Verification items for the finished model (mm, model axes). Coordinates: 2 decimals unless noted, no trailing zeros. Loops run counter-clockwise (first coordinate to the right, second up) from the corner with the lowest first, then second, coordinate; pieces in that order, holes last. Notation, with made-up numbers: (11.5, -29.5) - (49.5, -29.5) arc R34 cw to (49.5, 0.5) - close; hole circle Ø10 at (42.25, -5.5). An arc over 180 degrees is marked (long way). Answer as CSV lines item,"result". Start each with the question number.
1. Release check for a two-part mould opening along Y. For faces 1 (the cylindrical face through (265.014, -0.574, 1.972)), 2 (the cylindrical face through (-9.69, 0.42, 1.97)), 3 (the flat face through (125, 0, 4)) record: pulls with the +Y half, pulls with the -Y half, needs draft (parallel to the pull), parting line crosses it, or undercut.
2. Material ranges on line 1 (X direction, y = 0, z = 1.8); line 2 (X direction, y = 3, z = 2.95); line 3 (X direction, y = 8.5, z = 1), recorded low to high. Write a range as [from, to].
3. Cross-section at C-C (x = 250). Enter the section's corners in (y, z).
4. Cross-section at D-D (x = 136.5). Enter the section's corners in (y, z), plus the area to 3 significant figures.
5. Cross-section at A-A (x = 0). Enter the section's corners in (y, z).
6. Cross-section at B-B (z = 2.2). Enter the section's corners in (x, y).
7. Gauge pin test, flat ends, axial feed: P1, Ø2, axis at y = -2, z = 2.5, coming from the -X side; P2, Ø1, axis at y = 10.5, z = 0.5, coming from the +X side; P3, Ø1, axis at y = -8.5, z = 3.5, coming from the +X side. Record the tip position at first contact, or that the pin passes through.
```python
from build123d import *

# Parameters (mm, degrees)
SKETCH_1_R          = 9.7
SKETCH_1_R_2        = 1.5
EXTRUDE_1_DEPTH     = 4
SKETCH_3_R          = 0.8
CUT_EXTRUDE_1_DEPTH = 10


with BuildPart() as part:
    # 草图1 → 凸台-拉伸1 (new body)
    with BuildSketch(Plane.XY):
        with BuildLine():
            ThreePointArc((12.718684308, 6), (-14.062891969, 0), (12.718684308, -6))
            Line((12.718684308, -6), (236.224480753, -6))
            ThreePointArc((236.224480753, -6), (265.02547605, 0), (236.224480753, 6))
            Line((236.224480753, 6), (127.47158253, 6))
            ThreePointArc((127.47158253, 6), (124.47158253, 9), (121.47158253, 6))
            Line((121.47158253, 6), (12.718684308, 6))
        make_face()
        Circle(SKETCH_1_R, mode=Mode.SUBTRACT)
        with Locations((250, 0)):
            Circle(SKETCH_1_R, mode=Mode.SUBTRACT)
        with Locations((124.47158253, 6)):
            Circle(SKETCH_1_R_2, mode=Mode.SUBTRACT)
    extrude(amount=EXTRUDE_1_DEPTH)

    # 草图3 → 切除-拉伸1 (cut)
    with BuildSketch(Plane.XY.offset(4)):
        with Locations((9.7, 0)):
            Circle(SKETCH_3_R)
        with Locations((259.7, 0)):
            Circle(SKETCH_3_R)
    extrude(amount=-CUT_EXTRUDE_1_DEPTH, mode=Mode.SUBTRACT)


solid = part.part
```
Values follow:
1,face 1,"parting line crosses it"
1,face 2,"undercut"
1,face 3,"needs draft"
2,line 1,"x = [-14.06, -9.7], [10.5, 240.3], [260.5, 265.03]"
2,line 2,"x = [-13.74, -9.22], [9.22, 240.78], [259.22, 264.72]"
2,line 3,"x = [-11.2, -4.67], [4.67, 11.2], [122.81, 126.13], [237.61, 245.33], [254.67, 262.39]"
3,outline,"(-15.03, 0) - (-9.7, 0) - (-9.7, 4) - (-15.03, 4) - close; (9.7, 0) - (15.03, 0) - (15.03, 4) - (9.7, 4) - close"
4,outline,"(-6, 0) - (6, 0) - (6, 4) - (-6, 4) - close"
4,area,"48.0 mm²"
5,outline,"(-14.06, 0) - (-9.7, 0) - (-9.7, 4) - (-14.06, 4) - close; (9.7, 0) - (14.06, 0) - (14.06, 4) - (9.7, 4) - close"
6,outline,"(12.72, -6) - (236.22, -6) arc R15.03 ccw (long way) to (236.22, 6) - (127.47, 6) arc R3 ccw to (121.47, 6) - (12.72, 6) arc R14.06 ccw (long way) to start; hole (9.67, -0.8) arc R0.8 ccw (long way) to (9.67, 0.8) arc R9.7 ccw (long way) to start; hole circle Ø3 at (124.47, 6); hole (259.67, -0.8) arc R0.8 ccw (long way) to (259.67, 0.8) arc R9.7 ccw (long way) to start"
7,P1,"stops at x = -14.03"
7,P2,"stops at x = 261.21"
7,P3,"stops at x = 262.72"
